Verification items for the finished model (mm, model axes). Face numbers are marked on the shaded views. Coordinates: 2 decimals unless noted, no trailing zeros. Write each loop counter-clockwise with the first axis right and the second up, starting at its lowest first coordinate (ties: lowest second). Pieces come first, ordered by that corner, then holes. Notation, with made-up numbers: (56, 54) -> (83, 54) arc R32 cw to (83, 81) -> close; hole circle Ø5 at (19, 69). An arc over 180 degrees is marked (long way). Write item = value, one per line. Start each with the question number.
(1) Section check B-B (x = -30). Record the cut outline in (y, z), plus the area to 3 significant figures.
(2) Material ranges on probe 1 along Z at (x, y) = (0, 51); probe 2 along Y at (x, z) = (3, 460); probe 3 along Y at (x, z) = (0, 329.5), recorded low to high. Write a range as [from, to].
(3) Section check A-A (y = 0). Record the cut outline in (x, z), plus the area to 3 significant figures.
(4) Gauge pin test, flat ends, axial feed: pin 1 Ø5 at (y, z) = (-39, 301) entering from +X; pin 2 Ø12 at (x, z) = (24.5, 357.5) entering from +Y; pin 3 Ø1.5 at (x, z) = (16, 394.5) entering from +Y. Record the tip position at first contact, or that the pin passes through.
(5) Mould release check, pull along X, two halves, no side actions. Record for the marked faces 1 and 2: released by +X, released by -X, zero draft, split by the parting line, or undercut.
(6) Section check C-C (z = 361). Record the cut outline in (x, y), plus the area to 3 significant figures.
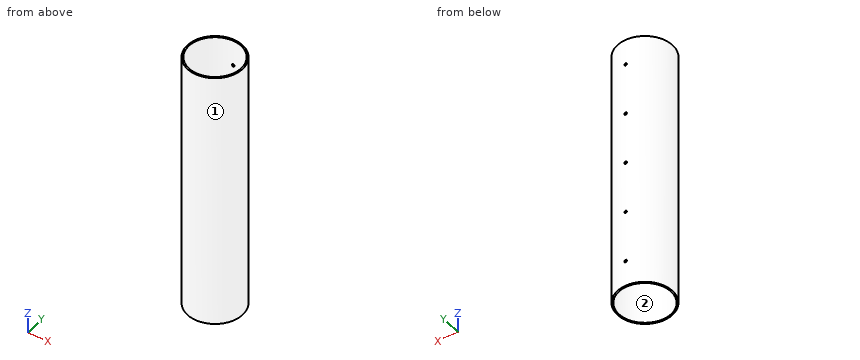
```python
from build123d import *

# Parameters (mm, degrees)
F0_R     = 53
F0_R_2   = 50
F1_DEPTH = 500
F3_D     = 5
F3_DEPTH = 53.001


with BuildPart() as f1:
    # F0 (on Top) → F1 (new body)
    with BuildSketch(Plane.XY):
        Circle(F0_R)
        Circle(F0_R_2, mode=Mode.SUBTRACT)
    extrude(amount=F1_DEPTH)

    # F3 (through all, one way)
    with BuildSketch(Plane.XZ):
        with Locations((0, 450), (0, 350), (0, 250), (0, 150), (0, 50)):
            Circle(F3_D / 2)
    extrude(amount=-F3_DEPTH, mode=Mode.SUBTRACT)


solid = f1.part
```
Response:
q1.outline = (-43.69, 0) -> (-40, 0) -> (-40, 500) -> (-43.69, 500) -> close; (40, 0) -> (43.69, 0) -> (43.69, 500) -> (40, 500) -> close
q1.area = 3,690 mm2
q2.probe_1 = [0, 47.5], [52.5, 147.5], [152.5, 247.5], [252.5, 347.5], [352.5, 447.5], [452.5, 500]
q2.probe_2 = [-52.92, -49.91], [49.91, 52.92]
q2.probe_3 = [-53, -50], [50, 53]
q3.outline = (-53, 0) -> (-50, 0) -> (-50, 500) -> (-53, 500) -> close; (50, 0) -> (53, 0) -> (53, 500) -> (50, 500) -> close
q3.area = 3,000 mm2
q4.pin_1 = 38.43
q4.pin_2 = 49.67
q4.pin_3 = 50.76
q5.face_1 = split by the parting line
q5.face_2 = undercut
q6.outline = circle Ø106 at (0, 0); hole circle Ø100 at (0, 0)
q6.area = 971 mm2
